Drawing for the job (mm, zero at the part's lowest x, y, z). A direction names the side the tool comes from. Give positions to 0.01 mm unless a question says otherwise; leave off trailing zeros. Order: outer loops, then holes, each group sorted by start corner. A loop starts at its lowest first (then second) coordinate and runs counter-clockwise, first axis right, second up. Notation, with made-up numbers: (20, -1) - (63, -1) arc R5 cw to (63, 5) - close; hole circle Ø4 at (26, 68). An arc over 180 degrees is marked (long way). Use a Markdown table: item, result. Add a question column.
(1) Mould opens along Y. For the marked faces 1, 2 and 3 say: +Y half, -Y half, draft (parallel to the pull), parting line (faces both ways), or undercut.
(2) Slice it at B-B (x = 11). Write the cut outline in (y, z).
(3) Slice it at C-C (z = 8.25). Write the cut outline in (x, y) (1 decimal).
(4) Slice it at D-D (y = 2). Write the cut outline in (x, z) (1 decimal).
(5) Flat gauge pins, fed straight in: pin 1 (2.5 mm diameter, centred on x = 34.5, z = 6, fed in from +Y); pin 2 (2.5 mm diameter, centred on y = 6.5, z = 4, fed in from -X); pin 3 (6.5 mm diameter, centred on x = 9.59, y = 9.66, fed in from +Z) (3 decimals); pin 4 (5 mm diameter, centred on y = 2.5, z = 8, fed in from +X). Where does each tip first touch, or does it go through?
(6) Slice it at A-A (y = 8.5). Write the cut outline in (x, z) (1 decimal).
(7) Wall check: line 1 (X direction, y = 4.5, z = 4.75) (1 decimal); line 2 (X direction, y = 6, z = 1.5); line 3 (Z direction, x = 6, y = 2). Give the ranges that are in metal, low to high.
(8) Which spindle directions (+Z, -Z, +X, -X, +Y, -Y) get a long thin tool onto all of the face, cutting with end or side? Do the marked faces 4, 5, 6 and 7. Say none if no direction does.
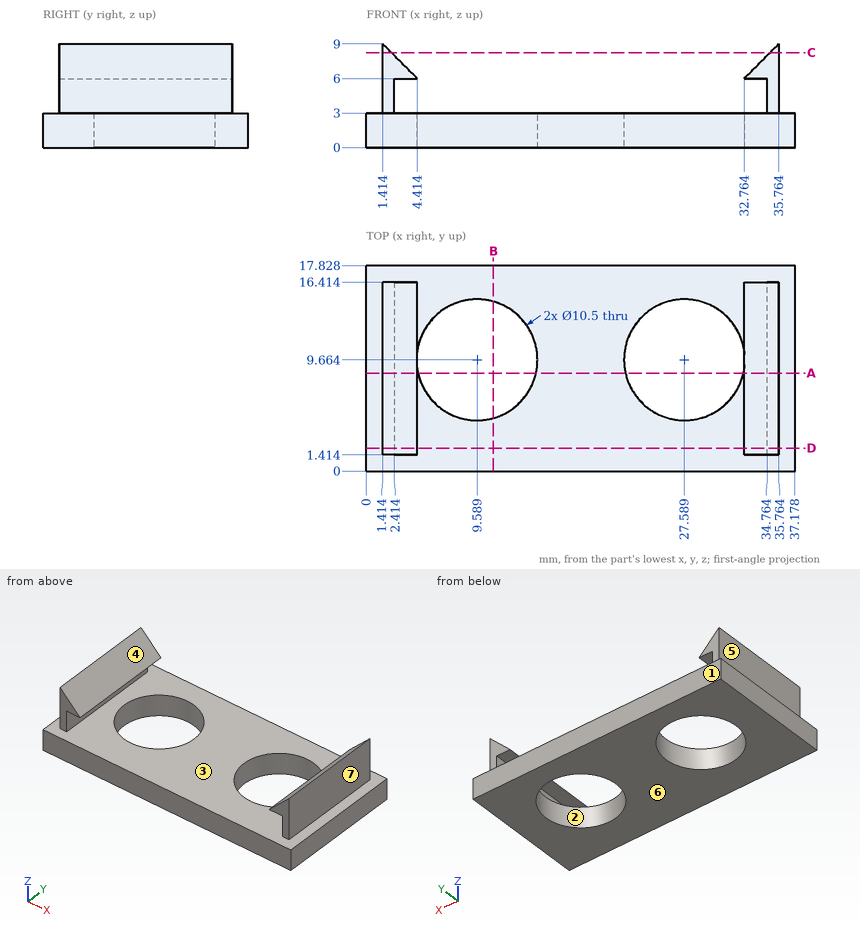
Solution:
| question | item | result |
|---|---|---|
| 1 | face 1 | +Y half |
| 1 | face 2 | undercut |
| 1 | face 3 | draft |
| 2 | outline | (0, 0) - (4.61, 0) - (4.61, 3) - (0, 3) - close; (14.72, 0) - (17.83, 0) - (17.83, 3) - (14.72, 3) - close |
| 3 | outline | (1.4, 1.4) - (2.2, 1.4) - (2.2, 16.4) - (1.4, 16.4) - close; (35, 1.4) - (35.8, 1.4) - (35.8, 16.4) - (35, 16.4) - close |
| 4 | outline | (0, 0) - (37.2, 0) - (37.2, 3) - (35.8, 3) - (35.8, 9) - (32.8, 6) - (34.8, 6) - (34.8, 3) - (2.4, 3) - (2.4, 6) - (4.4, 6) - (1.4, 9) - (1.4, 3) - (0, 3) - close |
| 5 | pin 1 | y = 16.41 |
| 5 | pin 2 | x = 0 |
| 5 | pin 3 | through |
| 5 | pin 4 | x = 35.76 |
| 6 | outline | (0, 0) - (4.5, 0) - (4.5, 3) - (2.4, 3) - (2.4, 6) - (4.4, 6) - (1.4, 9) - (1.4, 3) - (0, 3) - close; (14.7, 0) - (22.5, 0) - (22.5, 3) - (14.7, 3) - close; (32.7, 0) - (37.2, 0) - (37.2, 3) - (35.8, 3) - (35.8, 9) - (32.8, 6) - (34.8, 6) - (34.8, 3) - (32.7, 3) - close |
| 7 | line 1 | 1.4 to 2.4, 34.8 to 35.8 |
| 7 | line 2 | 0 to 5.83, 13.35 to 23.83, 31.35 to 37.18 |
| 7 | line 3 | 0 to 3 |
| 8 | face 4 | +Z, +Y, -Y |
| 8 | face 5 | +Z, -X, +Y, -Y |
| 8 | face 6 | -Z, +X, -X, +Y, -Y |
| 8 | face 7 | +Z, +X, +Y, -Y |
